Could you check a few things on this model? Use its own coordinates, in mm. A direction names the side the tool comes from. Coordinates: 2 decimals unless noted, no trailing zeros. Write each loop counter-clockwise with the first axis right and the second up, starting at its lowest first coordinate (ties: lowest second). Pieces come first, ordered by that corner, then holes. Notation, with made-up numbers: (79, 56) - (86, 56) arc R12 cw to (86, 71) - close; hole circle Ø9 at (-20, 82). An arc over 180 degrees is marked (long way). Answer as a JSON object with one key per item and string values. Group by question number.
1) If we section it at D-D (z = -10): Write out the boundary of the cut face in (x, y), plus the area to 3 significant figures.
2) If we section it at C-C (z = -18.5): Write out the boundary of the cut face in (x, y).
3) If we section it at B-B (y = 59): Write out the boundary of the cut face in (x, z), plus the area to 3 significant figures.
4) If we section it at A-A (x = -24.5): Write out the boundary of the cut face in (y, z), plus the area to 3 significant figures.
5) Will this pin go through, and if not, where does the flat tip stop? pin 1 Ø4 at (x, z) = (0, 0) entering from +Y.
6) Please list where these lines run through material, in increasing order: line 1 along X through (y, z) = (2, 0); line 2 along X through (y, z) = (121, 18.5); line 3 along Z through (x, y) = (0, 1.45).
7) On a 3-axis mill with a long thin cutter (end or side, diameter ignored), from which of +Z, -Z, +X, -X, +Y, -Y can I reach the whole of each face in a straight line? I mean faces 1 (the flat face through (-4, 130, 34)), 2 (the flat face through (-1, 66, 31.5)). Say none if no direction works.
8) We'd pull the mould along X, two halves only. Please class faces 3 (the flat face through (55, 64, 0)), 4 (the flat face through (-1, 3.5, 7)), 5 (the flat face through (-1, 0, -8)): released by +X, released by -X, zero draft, split by the parting line, or undercut.
```python
from build123d import *

# Parameters (mm, degrees)
CROQUIS1_W                 = 110
CROQUIS1_H                 = 70
SALIENTE_EXTRUIR3_DEPTH    = 130
VACIADO4_T                 = -3.5
CORTAR_EXTRUIR4_REACH      = 147.43
CROQUIS2_R                 = 6
CROQUIS2_R_2               = 1.5
CORTAR_EXTRUIR8_DEPTH      = 174.853386507
CORTAR_EXTRUIR8_DEPTH_BACK = 174.853386507


with BuildPart() as part:
    # Croquis1 → Saliente-Extruir3 (new body)
    with BuildSketch(Plane(origin=(0, 0, 0), x_dir=(1, 0, 0), z_dir=(0, 1, 0))):
        Rectangle(CROQUIS1_W, CROQUIS1_H)
    extrude(amount=SALIENTE_EXTRUIR3_DEPTH)

    # Vaciado4
    vaciado4_openings = [part.faces().sort_by_distance(p)[0] for p in [
        (0, 130, 0),
    ]]
    offset(amount=VACIADO4_T, openings=vaciado4_openings, kind=Kind.INTERSECTION)

    # Croquis2 → Cortar-Extruir4 (cut, up to next)
    with BuildSketch(Plane(origin=(0, 0, 0), x_dir=(1, 0, 0), z_dir=(0, 1, 0)), mode=Mode.PRIVATE) as cortar_extruir4_sk1:
        with Locations(Location((-24.5, 0, 0), (0, 0, 270))):
            Circle(CROQUIS2_R)
    cortar_extruir4_tool1 = extrude(cortar_extruir4_sk1.sketch, amount=CORTAR_EXTRUIR4_REACH, mode=Mode.PRIVATE) & part.part
    # Croquis2 → Cortar-Extruir4 (cut, up to next)
    with BuildSketch(Plane(origin=(0, 0, 0), x_dir=(1, 0, 0), z_dir=(0, 1, 0)), mode=Mode.PRIVATE) as cortar_extruir4_sk2:
        with Locations(Location((24.5, 0, 0), (0, 0, 270))):
            Circle(CROQUIS2_R)
    cortar_extruir4_tool2 = extrude(cortar_extruir4_sk2.sketch, amount=CORTAR_EXTRUIR4_REACH, mode=Mode.PRIVATE) & part.part
    # Croquis2 → Cortar-Extruir4 (cut, up to next)
    with BuildSketch(Plane(origin=(0, 0, 0), x_dir=(1, 0, 0), z_dir=(0, 1, 0)), mode=Mode.PRIVATE) as cortar_extruir4_sk3:
        with Locations(Location((0, 0, 0), (0, 0, 270))):
            Circle(CROQUIS2_R_2)
    cortar_extruir4_tool3 = extrude(cortar_extruir4_sk3.sketch, amount=CORTAR_EXTRUIR4_REACH, mode=Mode.PRIVATE) & part.part
    add(cortar_extruir4_tool1.solids().sort_by_distance((-24.5, 0, 0))[0], mode=Mode.SUBTRACT)
    add(cortar_extruir4_tool2.solids().sort_by_distance((24.5, 0, 0))[0], mode=Mode.SUBTRACT)
    add(cortar_extruir4_tool3.solids().sort_by_distance((0, 0, 0))[0], mode=Mode.SUBTRACT)

    # Croquis3 → Cortar-Extruir8 (cut, two sides: drawn at the far end of the back side and taken through both)
    with BuildSketch(Plane(origin=(55, 0, 0), x_dir=(0, 0, -1), z_dir=(1, 0, 0)).offset(-CORTAR_EXTRUIR8_DEPTH_BACK)):
        with BuildLine():
            Line((-15.212730717, 3.5), (14.783786757, 3.5))
            ThreePointArc((14.783786757, 3.5), (10.390898479, 14.105370459), (-0.21447198, 18.498258737))
            ThreePointArc((-0.21447198, 18.498258737), (-10.819842439, 14.105370459), (-15.212730717, 3.5))
        make_face()
    extrude(amount=CORTAR_EXTRUIR8_DEPTH + CORTAR_EXTRUIR8_DEPTH_BACK, mode=Mode.SUBTRACT)


solid = part.part
```
Here are the results:
{
 "1": {"outline": "(-55, 0) - (55, 0) - (55, 3.5) - (-55, 3.5) - close; (-55, 14.48) - (-51.5, 14.48) - (-51.5, 130) - (-55, 130) - close; (51.5, 14.48) - (55, 14.48) - (55, 130) - (51.5, 130) - close", "area": "1,190 mm²"},
 "2": {"outline": "(-55, 0) - (55, 0) - (55, 130) - (51.5, 130) - (51.5, 3.5) - (-51.5, 3.5) - (-51.5, 130) - (-55, 130) - close"},
 "3": {"outline": "(-55, -35) - (55, -35) - (55, 35) - (-55, 35) - close; hole (-51.5, -31.5) - (51.5, -31.5) - (51.5, 31.5) - (-51.5, 31.5) - close", "area": "1,210 mm²"},
 "4": {"outline": "(0, -35) - (130, -35) - (130, -31.5) - (3.5, -31.5) - (3.5, -6) - (0, -6) - close; (0, 6) - (3.5, 6) - (3.5, 31.5) - (130, 31.5) - (130, 35) - (0, 35) - close", "area": "1,090 mm²"},
 "5": {"pin 1": "stops at y = 3.5"},
 "6": {"line 1": "x = -55 to -30.5, -18.5 to -1.5, 1.5 to 18.5, 30.5 to 55", "line 2": "x = -55 to -51.5, 51.5 to 55", "line 3": "z = -35 to -1.5, 1.5 to 35"},
 "7": {"face 1": "+Z, -Z, +X, -X, +Y", "face 2": "+Y"},
 "8": {"face 3": "released by +X", "face 4": "undercut", "face 5": "zero draft"}
}
